Can you work these out from the model? Positions are in its coordinate system, mm. A direction names the side the tool comes from. Give positions to 0.01 mm unless a question says otherwise; leave off trailing zeros. Loops run counter-clockwise (first coordinate to the right, second up) from the corner with the lowest first, then second, coordinate; pieces in that order, holes last.
from build123d import *

# Parameters (mm, degrees)
F1_DEPTH = 12.7
F2_W     = 3.6453269422
F2_H     = 2.4501346052
F3_DEPTH = 5.08
F4_DEPTH = 5.08


with BuildPart() as f1:
    # F0 (on Top) → F1 (new body)
    with BuildSketch(Plane.XY):
        Polygon((6.5544429235, 37.8296226263), (6.5544429235, 41.3456484675), (3.76586942, 39.5876355469), (3.76586942, 33.586140722), (12.4953174964, 24.6142074466), (15.2838900685, 25.9478744119), (14.313952066, 27.5240242481), (14.313952066, 30.0701130182), (20.9822803736, 22.5530881435), (14.313952066, 15.521033667), (11.8891056627, 14.0661261976), (15.7688595355, 11.3987950608), (17.1025265008, 7.1553131565), (19.0424025059, 11.3987950608), (25.4682451487, 18.9158190042), (32.7427871525, 11.3987950608), (34.925147891, 6.791586522), (36.0163263977, 11.3987950608), (38.9261469245, 14.0661261976), (37.1075086296, 15.521033667), (30.0754550844, 22.5530881435), (37.1075086296, 30.0701130182), (37.1075086296, 27.5240242481), (35.8950868249, 25.9478744119), (38.5624170303, 24.6142074466), (47.5343503058, 33.586140722), (47.5343503058, 39.5876355469), (44.6245335042, 41.3456484675), (44.6245335042, 37.8296226263), (37.1075086296, 38.7995615602), (34.0764522552, 41.3456484675), (31.1666354537, 41.3456484675), (34.0764522552, 38.7995615602), (34.0764522552, 35.0410491228), (30.0754550844, 30.5550824851), (25.5894884467, 35.0410491228), (20.9822803736, 30.5550824851), (17.2237679362, 35.0410491228), (17.2237679362, 38.7995615602), (20.0123414397, 41.3456484675), (17.2237679362, 41.3456484675), (14.313952066, 38.7995615602), align=None)
        Polygon((24.5242901146, 30.8284908533), (25.5894884467, 31.9072976708), (26.8167555332, 30.8284908533), (25.5894884467, 29.5136924833), align=None, mode=Mode.SUBTRACT)
    extrude(amount=F1_DEPTH)

    # F2 (on face) → F3 (cut)
    with BuildSketch(Plane.XY.offset(12.7)):
        Polygon((7.0490693162, 37.8914509439), (6.5544429235, 37.8296226263), (6.0410341248, 35.2296121418), (14.313952066, 27.5240242481), (14.313952066, 30.0701130182), (20.9822803736, 22.5530881435), (14.313952066, 15.521033667), (19.0424025059, 11.3987950608), (25.4682451487, 18.9158190042), (32.7427871525, 11.3987950608), (37.1075086296, 15.521033667), (30.0754550844, 22.5530881435), (37.1075086296, 30.0701130182), (37.1075086296, 27.5240242481), (36.5012977272, 26.73594933), (44.8912195861, 34.5637351274), (44.6245335042, 37.8296226263), (37.1075086296, 38.7995615602), (37.1075086296, 30.5685326457), (34.6490368247, 28.4877605736), (34.6490368247, 30.5685326457), (34.6490368247, 38.7995615602), (34.0764522552, 38.7995615602), (34.0764522552, 35.0410491228), (30.0754550844, 30.5550824851), (29.8693068326, 30.761230737), (21.7151734978, 22.8682607412), (20.5283816904, 24.3646502495), (25.694264099, 29.3949842453), (25.5894884467, 29.5136924833), (25.4240528691, 29.7178933549), (24.0751728415, 28.4491963685), (21.2630781019, 30.8284908533), (20.9822803736, 30.5550824851), (17.2237679362, 35.0410491228), (17.2237679362, 38.7995615602), (16.6432019323, 38.4291112423), (16.8820619583, 28.1179565936), (14.313952066, 30.6153800339), (14.313952066, 38.7995615602), align=None)
        Polygon((15.5932606215, 15.7401643943), (21.7151734978, 21.8692570925), (23.0203711557, 20.550046149), (16.8623554934, 14.4574438554), align=None, mode=Mode.SUBTRACT)
        Polygon((17.6451402405, 13.9573783364), (23.711329326, 20.1660916209), (24.9279786679, 18.9555015123), (18.8057093955, 12.8025891205), align=None, mode=Mode.SUBTRACT)
        Polygon((32.7832475305, 12.346426025), (22.4977247417, 22.5807242095), (23.8481555134, 23.8528680056), (34.1030471027, 13.4878745303), align=None, mode=Mode.SUBTRACT)
        Polygon((26.2261033058, 22.6549040526), (27.4469424039, 23.696700111), (35.9935723245, 15.4675748199), (34.6024334431, 14.1477743164), align=None, mode=Mode.SUBTRACT)
        Polygon((17.4691583961, 27.6918299496), (17.4691583961, 30.1007553935), (21.482238546, 26.135975495), (20.2486850321, 24.7733257711), align=None, mode=Mode.SUBTRACT)
        Polygon((17.4691583961, 31.1430785805), (17.4691583961, 33.8531173766), (23.445142433, 28.0161090195), (22.0553781837, 26.7189964652), align=None, mode=Mode.SUBTRACT)
        Polygon((7.5238011777, 34.6592962742), (10.6979301199, 34.5851331949), (10.4632368311, 32.0025421679), align=None, mode=Mode.SUBTRACT)
        Polygon((6.9207791239, 35.0040383637), (6.9207791239, 37.3774655163), (10.6979301199, 37.3774655163), (10.6979301199, 35.1172611117), align=None, mode=Mode.SUBTRACT)
        Polygon((13.6304246262, 28.7970686331), (11.0295182094, 31.0556814075), (11.1747216433, 37.3774655163), (13.784497045, 37.3774655163), align=None, mode=Mode.SUBTRACT)
        Polygon((27.9130805284, 24.2891721427), (29.262598604, 25.6057772785), (30.5133741349, 24.2891721427), (29.3284300715, 23.1042280793), align=None, mode=Mode.SUBTRACT)
        Polygon((30.9950727969, 24.886559695), (29.7354832292, 26.1461511254), (33.9365452528, 29.8445243388), (33.9365452528, 27.5129415095), align=None, mode=Mode.SUBTRACT)
        Polygon((24.3253335357, 24.3550017476), (33.9036285877, 34.1307893395), (33.9365452528, 31.2342606485), (25.5894884467, 22.9456070811), align=None, mode=Mode.SUBTRACT)
        Polygon((37.6231558621, 30.7271517813), (37.6231558621, 37.5519581139), (40.1610732079, 37.5519581139), (40.1610732079, 30.7271517813), (37.6231558621, 28.4877605736), align=None, mode=Mode.SUBTRACT)
        Polygon((40.6824201345, 34.5267690718), (43.7329895794, 34.5558524132), (40.6824201345, 31.5891802311), align=None, mode=Mode.SUBTRACT)
        with Locations((42.5050836056, 36.3268908113)):
            Rectangle(F2_W, F2_H, mode=Mode.SUBTRACT)
    extrude(amount=-F3_DEPTH, mode=Mode.SUBTRACT)

    # F4 (cut): a face of the model
    f4_faces = [f1.faces().sort_by_distance(p)[0] for p in [
        (25.6298789879, 27.4747864978, 0),
    ]]
    extrude(f4_faces, amount=-F4_DEPTH, mode=Mode.SUBTRACT)


solid = f1.part
(1) Will these pins go through, and if not, where does the flat tip stop? P1, Ø4, axis at x = 25.5, z = 6, coming from the -Y side; P2, Ø1.9, axis at x = 9.5, z = 9.5, coming from the +Y side; P3, Ø3, axis at x = 12, z = 9, coming from the -Y side.
Returned:
P1: stops at y = 16.61
P2: stops at y = 37.38
P3: stops at y = 12.96
(2) Suppose I cut it at C-C on x = 28.5. List the corners of the cut face in (y, z) for me.
Returned:
outline: (15.78, 5.08) - (32.13, 5.08) - (32.13, 12.7) - (29.44, 12.7) - (29.44, 7.62) - (28.62, 7.62) - (28.62, 12.7) - (25.84, 12.7) - (25.84, 7.62) - (24.86, 7.62) - (24.86, 12.7) - (23.8, 12.7) - (23.8, 7.62) - (22.68, 7.62) - (22.68, 12.7) - (20.35, 12.7) - (20.35, 7.62) - (19.15, 7.62) - (19.15, 12.7) - (16.61, 12.7) - (16.61, 7.62) - (15.78, 7.62) - close
(3) Suppose I cut it at B-B on z = 10.25. Give the number of separate pieces and of enclosed holes in the cut face, plus the area to 3 significant figures.
Returned:
separate pieces: 22
enclosed holes: 0
area: 452 mm2
(4) Please list where these lines run through material, in increasing order: probe 1 along Y at (x, z) = (28, 10.5); probe 2 along X at (y, z) = (21.5, 8.75); probe 3 along Y at (x, z) = (25, 9.5).
Returned:
probe 1: y = 17.11 to 19.66, 20.85 to 23.16, 24.22 to 24.37, 25.34 to 28.11, 28.95 to 32.63
probe 2: x = 21.35 to 22.08, 23.58 to 26.18, 27.36 to 29.73
probe 3: y = 20.09 to 22.69, 23.6 to 25.04, 26.05 to 28.72, 29.32 to 30.24, 31.31 to 34.47
(5) Suppose I cut it at D-D on x = 42.5. List the corners of the cut face in (y, z) for me.
Returned:
outline: (28.55, 5.08) - (38.1, 5.08) - (38.1, 7.62) - (37.55, 7.62) - (37.55, 12.7) - (35.1, 12.7) - (35.1, 7.62) - (34.54, 7.62) - (34.54, 12.7) - (33.36, 12.7) - (33.36, 7.62) - (32.33, 7.62) - (32.33, 12.7) - (28.55, 12.7) - close
(6) Thinking about a two-plate mould opening in X: for faces 6 (the flat face through (14.314, 29, 6)), 7 (the flat face through (21.13, 23.606, 10.196)), 8 (the flat face through (9, 36, 12.7)), which applies, pulls with the +X half, pulls with the -X half, needs draft (parallel to the pull), parting line crosses it, or undercut?
Returned:
face 6: undercut
face 7: pulls with the -X half
face 8: needs draft
(7) Which directions (+Z, -Z, +X, -X, +Y, -Y) give clear straight access to the entire face, cutting with the end or side of a thin tool? Please do faces 1 (the flat face through (27.86, 32.77, 8.84)), 2 (the flat face through (33.542, 26.259, 6.332)), 3 (the flat face through (27.712, 17.392, 10.196)), 4 (the flat face through (33, 41.346, 9)), 5 (the flat face through (37.623, 33, 10)).
Returned:
face 1: +Z, -Z, +Y
face 2: +Z, -Z
face 3: +Z
face 4: +Z, -Z, +X, -X, +Y
face 5: +Z, +Y
(8) Suppose I cut it at A-A on x = 13. List the corners of the cut face in (y, z) for me, plus the area to 3 significant figures.
Returned:
outline: (13.3, 5.08) - (14.73, 5.08) - (14.73, 12.7) - (13.3, 12.7) - close; (24.86, 5.08) - (38.64, 5.08) - (38.64, 7.62) - (37.38, 7.62) - (37.38, 12.7) - (29.34, 12.7) - (29.34, 7.62) - (28.75, 7.62) - (28.75, 12.7) - (24.86, 12.7) - close
area: 106 mm2
